Check sheet for the drawn part. Datum: minimum x, y, z corner. Units: mm. Give positions to 0.01 mm unless a question says otherwise; leave off trailing zeros. Order: outer loops, then holes, each group sorted by start corner. A loop starts at its lowest first (then second) coordinate and runs counter-clockwise, first axis right, second up. Notation, with made-up numbers: M 70,80 L 98,80 A15 cw 98,109 Z; hole C -6,45.25 d11. An arc over 180 degrees is marked long. Put each result on its own line as item: value. Start each with the question number.
Q1. Go/stop test with a flat-tipped pin: pin 1 (5 mm diameter, centred on x = 141, y = 37.5, fed in from +Z). Record where the tip stops, or that it passes through.
Q2. Section check B-B on y = 8. Record the cut outline in (x, z), then the cut area to 4 significant figures.
Q3. Section check A-A on z = 948. Record the cut outline in (x, y), then the cut area to 3 significant figures.
Q4. Material ranges on L1, parallel to X at y = 5.5, z = 781; L2, parallel to Z at x = 163.5, y = 22, recorded low to high.
Q5. Section check C-C on x = 161. Record the cut outline in (y, z).
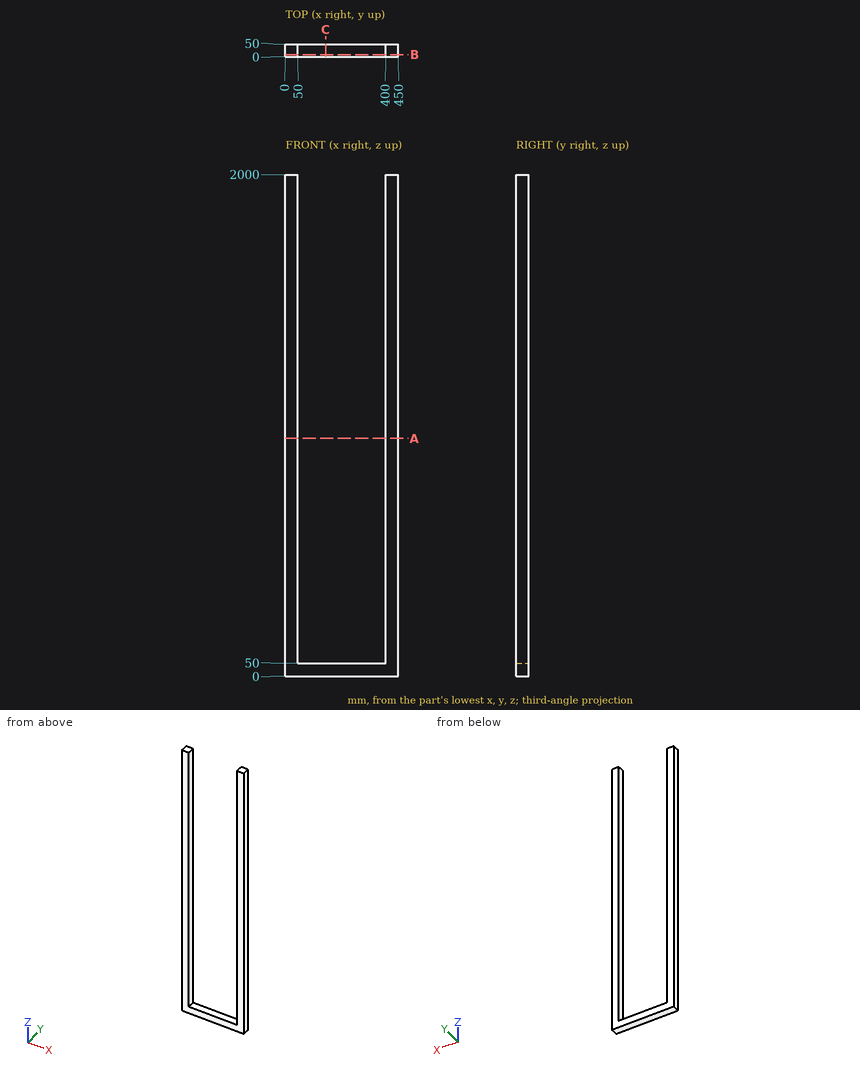
Results found:
1. pin 1: stops at z = 50
2. outline: M 0,0 L 450,0 L 450,2000 L 400,2000 L 400,50 L 50,50 L 50,2000 L 0,2000 Z
2. area: 217,500 mm^2
3. outline: M 0,0 L 50,0 L 50,50 L 0,50 Z; M 400,0 L 450,0 L 450,50 L 400,50 Z
3. area: 5,000 mm^2
4. L1: x = 0 to 50, 400 to 450
4. L2: z = 0 to 50
5. outline: M 0,0 L 50,0 L 50,50 L 0,50 Z
